from build123d import *

# Parameters (mm, degrees)
SKETCH1_R               = 10
BOSS_EXTRUDE1_DEPTH     = 900
SKETCH2_R               = 8
CUT_EXTRUDE1_DEPTH      = 40
CUT_EXTRUDE2_START      = -40
SKETCH3_R               = 8
CUT_EXTRUDE2_DEPTH      = 40
CUT_EXTRUDE3_DEPTH      = 40
CUT_EXTRUDE3_DEPTH_BACK = 40
SKETCH4_R               = 4


with BuildPart() as part:
    # Sketch1 → Boss-Extrude1 (new body)
    with BuildSketch(Plane.YZ):
        with Locations(Location((0, 0, 0), (0, 0, 270))):
            Circle(SKETCH1_R)
    extrude(amount=BOSS_EXTRUDE1_DEPTH)

    # Sketch2 → Cut-Extrude1 (cut)
    with BuildSketch(Plane.YZ.offset(900)):
        with Locations(Location((0, 0, 0), (0, 0, 270))):
            Circle(SKETCH2_R)
    extrude(amount=-CUT_EXTRUDE1_DEPTH, mode=Mode.SUBTRACT)

    # Sketch3 → Cut-Extrude2 (cut)
    with BuildSketch(Plane(origin=(0, 0, 0), x_dir=(0, -1, 0), z_dir=(-1, 0, 0)).offset(CUT_EXTRUDE2_START)):
        with Locations(Location((0, 0, 0), (0, 0, 270))):
            Circle(SKETCH3_R)
    extrude(amount=CUT_EXTRUDE2_DEPTH, mode=Mode.SUBTRACT)

    # Sketch4 → Cut-Extrude3 (cut, two sides: drawn at the far end of the back side and taken through both)
    with BuildSketch(Plane(origin=(0, 0, 0), x_dir=(-1, 0, 0), z_dir=(0, 1, 0)).offset(-CUT_EXTRUDE3_DEPTH_BACK)):
        with Locations(Location((-130, 0, 0), (0, 0, 270))):
            Circle(SKETCH4_R)
        with Locations(Location((-770, 0, 0), (0, 0, 270))):
            Circle(SKETCH4_R)
    extrude(amount=CUT_EXTRUDE3_DEPTH + CUT_EXTRUDE3_DEPTH_BACK, mode=Mode.SUBTRACT)


solid = part.part
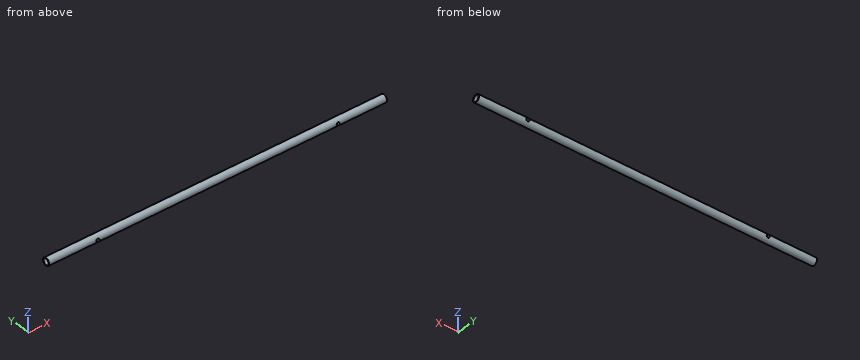
Source: CAD feature listing. Evaluate the final solid. Frame: model axes, mm. Round coordinates to 2 decimals unless told otherwise and drop trailing zeros. Loops run counter-clockwise (first coordinate to the right, second up) from the corner with the lowest first, then second, coordinate; pieces in that order, holes last. Notation, with made-up numbers: M 1,7.25 L 30,7.25 A23 ccw 30,42.25 Z; hole C -26.5,22.5 d11. An arc over 180 degrees is marked long. Answer as CSV lines item,"result".
Q1. Contact query for flat-ended pins moving along their axis: pin 1 (2 mm diameter, centred on x = 510, z = -5.5, fed in from +Y); pin 2 (6 mm diameter, centred on y = -2.5, z = -1, fed in from -X); pin 3 (1.5 mm diameter, centred on x = 150.5, z = -8, fed in from -Y). Output: stop coordinate, or through.
Verdict:
pin 1,"stops at y = 8.93"
pin 2,"stops at x = 40"
pin 3,"stops at y = -6.89"
Q2. Line query: line 1 along X through (y, z) = (5.5, 0); line 2 along Y through (x, z) = (16.5, 0); line 3 along X through (y, z) = (2.25, 3). Output: solid intervals per line, ascending.
Verdict:
line 1,"x = 40 to 126, 134 to 766, 774 to 860"
line 2,"y = -10 to -8, 8 to 10"
line 3,"x = 40 to 127.35, 132.65 to 767.35, 772.65 to 860"
Q3. Cut plane A-A (y = 0). Return the cut outline in (x, z).
Verdict:
outline,"M 0,-10 L 900,-10 L 900,-8 L 860,-8 L 860,8 L 900,8 L 900,10 L 0,10 L 0,8 L 40,8 L 40,-8 L 0,-8 Z; hole C 130,0 d8; hole C 770,0 d8"
Q4. Cut plane C-C (x = 323.5). Return the cut outline in (y, z), plus the area to 3 significant figures.
Verdict:
outline,"C 0,0 d20"
area,"314 mm^2"
Q5. Cut plane B-B (z = -0.75). Return the cut outline in (x, y), plus the area to 3 significant figures.
Verdict:
outline,"M 0,-9.97 L 126.07,-9.97 L 126.07,9.97 L 0,9.97 L 0,7.96 L 40,7.96 L 40,-7.96 L 0,-7.96 Z; M 133.93,-9.97 L 766.07,-9.97 L 766.07,9.97 L 133.93,9.97 Z; M 773.93,-9.97 L 900,-9.97 L 900,-7.96 L 860,-7.96 L 860,7.96 L 900,7.96 L 900,9.97 L 773.93,9.97 Z"
area,"16,400 mm^2"
